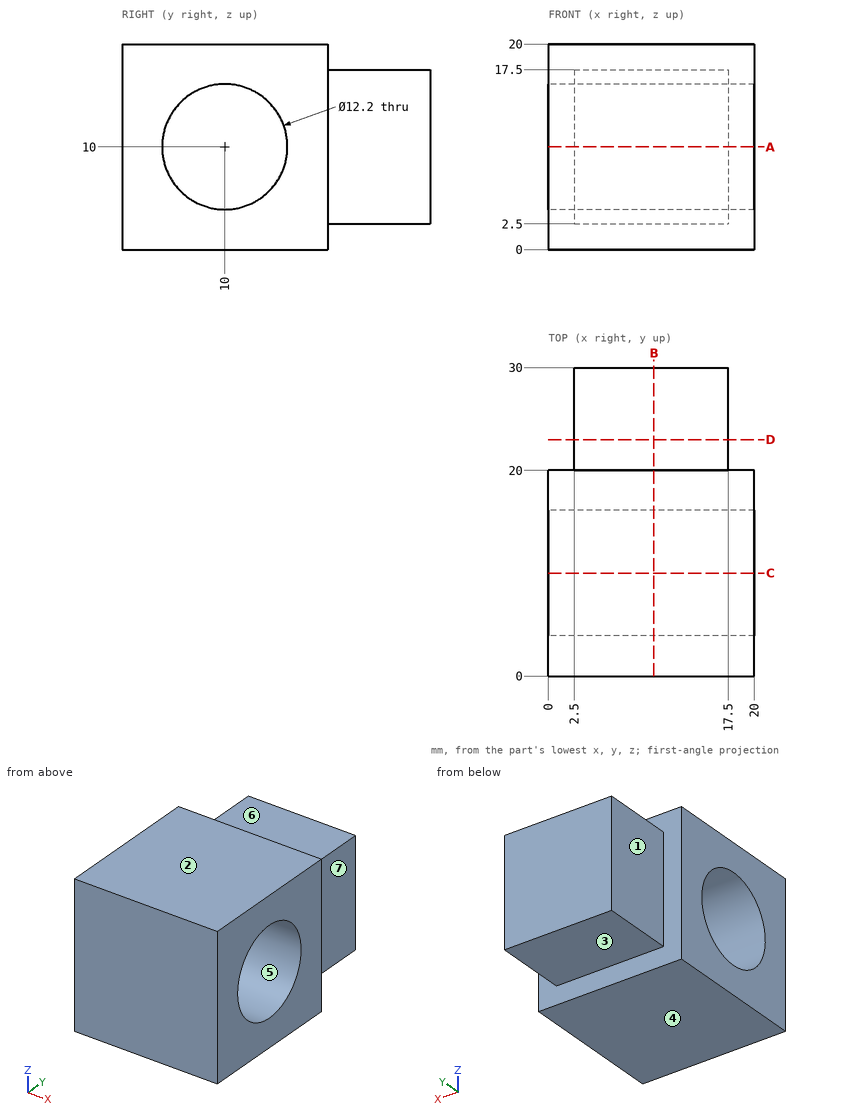
Design review of the part shown in the three views and the two pictorial views. Dimensions are in mm from the part's minimum x, y and z. A direction names the side the tool comes from. Round coordinates to 2 decimals unless told otherwise and drop trailing zeros. Loops run counter-clockwise (first coordinate to the right, second up) from the corner with the lowest first, then second, coordinate; pieces in that order, holes last.
(1) We need section C-C (y = 10). Give the boundary of the cut face in (x, z).
Returned:
outline: (0, 0) - (20, 0) - (20, 3.9) - (0, 3.9) - close; (0, 16.1) - (20, 16.1) - (20, 20) - (0, 20) - close
(2) Clearance check with flat-ended pins moving along their axes: P1, Ø5, axis at x = 11, y = 26, coming from the +Z side; P2, Ø12, axis at x = 7.5, y = 13, coming from the -Z side; P3, Ø1.5, axis at x = 16, y = 26, coming from the -Z side; P4, Ø11, axis at y = 10, z = 10, coming from the +X side. State where each tip first meets the part, or that it passes through.
Returned:
P1: stops at z = 17.5
P2: stops at z = 0
P3: stops at z = 2.5
P4: passes through
(3) We need section A-A (z = 10). Give the boundary of the cut face in (x, y).
Returned:
outline: (0, 0) - (20, 0) - (20, 3.9) - (0, 3.9) - close; (0, 16.1) - (20, 16.1) - (20, 20) - (17.5, 20) - (17.5, 30) - (2.5, 30) - (2.5, 20) - (0, 20) - close
(4) Wall thickness on line 1 along Y through (x, z) = (7.75, 10); line 2 along X through (y, z) = (28, 4.75); line 3 along Z through (x, y) = (9, 11.5): over which ranges is each line inside the solid? List them lowest first.
Returned:
line 1: y = 0 to 3.9, 16.1 to 30
line 2: x = 2.5 to 17.5
line 3: z = 0 to 4.09, 15.91 to 20
(5) We need section D-D (y = 23). Give the boundary of the cut face in (x, z), plus the area to 3 significant figures.
Returned:
outline: (2.5, 2.5) - (17.5, 2.5) - (17.5, 17.5) - (2.5, 17.5) - close
area: 225 mm2
(6) We need section B-B (x = 10.25). Give the boundary of the cut face in (y, z).
Returned:
outline: (0, 0) - (20, 0) - (20, 2.5) - (30, 2.5) - (30, 17.5) - (20, 17.5) - (20, 20) - (0, 20) - close; hole circle Ø12.2 at (10, 10)
(7) Mouldability with a two-part tool opening along Z and no side actions: class the marked faces 4, 5, 6 and 7 as released by +Z, released by -Z, zero draft, split by the parting line, or undercut.
Returned:
face 4: released by -Z
face 5: undercut
face 6: released by +Z
face 7: zero draft
(8) Tool access review of the marked faces 1, 2 and 3: name each direction out of +Z, -Z, +X, -X, +Y, -Y from which nothing blocks a thin tool from reaching the whole face with its end or side.
Returned:
face 1: +Z, -Z, -X, +Y
face 2: +Z, +X, -X, +Y, -Y
face 3: -Z, +X, -X, +Y
